from build123d import *

# Parameters (mm, degrees)
BOSS_EXTRUDE1_DEPTH = 100


with BuildPart() as part:
    # Sketch1 → Boss-Extrude1 (new body)
    with BuildSketch(Plane.XY):
        with BuildLine():
            Line((0, 0), (11, 0))
            Line((11, 0), (11, -0.9))
            Line((11, -0.9), (9.5, -0.9))
            ThreePointArc((9.5, -0.9), (9.128025612, -1.798025612), (8.23, -2.17))
            Line((8.23, -2.17), (8.23, -3.07))
            Line((8.23, -3.07), (12.415281374, -3.07))
            Line((12.415281374, -3.07), (13.949747468, -1.535533906))
            Line((13.949747468, -1.535533906), (10.414213562, 2))
            Line((10.414213562, 2), (0.585786438, 2))
            Line((0.585786438, 2), (-2.814747468, -1.400533906))
            Line((-2.814747468, -1.400533906), (-1.145281374, -3.07))
            Line((-1.145281374, -3.07), (2.77, -3.07))
            Line((2.77, -3.07), (2.77, -2.17))
            ThreePointArc((2.77, -2.17), (1.871974388, -1.798025612), (1.5, -0.9))
            Line((1.5, -0.9), (0, -0.9))
            Line((0, -0.9), (0, 0))
        make_face()
    extrude(amount=BOSS_EXTRUDE1_DEPTH)


solid = part.part
Geometry: final body of the model. Coordinates: model frame, mm. Round coordinates to 2 decimals unless told otherwise and drop trailing zeros. Loops run counter-clockwise (first coordinate to the right, second up) from the corner with the lowest first, then second, coordinate; pieces in that order, holes last.
Q1. Material intervals for L1, parallel to Y at x = 3.5, z = 46; L2, parallel to X at y = -0.75, z = 58; L3, parallel to X at y = -2.65, z = 77, sorted ascending.
Q2. Pin query (flat end, axial travel): P1, Ø1, axis at x = 7.5, z = 67.5, coming from the -Y side; P2, Ø0.7, axis at y = -2.5, z = 74.5, coming from the -X side; P3, Ø1.5, axis at y = -2.5, z = 83, coming from the +X side. Return the tip coordinate at first contact, or that it passes through.
Q3. Section A-A on z = 9. Return loops of the section in (x, y).
Q4. Section B-B on x = 5.25. Return loops of the section in (y, z), plus the area to 3 significant figures.
Q5. Section C-C on y = 0.8. Return loops of the section in (x, z), plus the area to 3 significant figures.
Q6. Pull-direction query (Y, two-part tool) for faces 1 (the flat face through (5, 1, 100)), 2 (the flat face through (13.172, -2.314, 49.3)), 3 (the flat face through (-1.091, 0.324, 49.3)), 4 (the flat face through (5, 0, 49)); classes: released by +Y, released by -Y, zero draft, split by the parting line, or undercut.
Evaluation:
1. L1: y = 0 to 2
1. L2: x = -2.16 to 0, 11 to 13.16
1. L3: x = -1.57 to 2.77, 8.23 to 12.84
2. P1: stops at y = 0
2. P2: stops at x = -2.07
2. P3: stops at x = 13.74
3. outline: (-2.81, -1.4) - (-1.15, -3.07) - (2.77, -3.07) - (2.77, -2.17) arc R1.27 cw to (1.5, -0.9) - (0, -0.9) - (0, 0) - (11, 0) - (11, -0.9) - (9.5, -0.9) arc R1.27 cw to (8.23, -2.17) - (8.23, -3.07) - (12.42, -3.07) - (13.95, -1.54) - (10.41, 2) - (0.59, 2) - close
4. outline: (0, 0) - (2, 0) - (2, 100) - (0, 100) - close
4. area: 200 mm2
5. outline: (-0.61, 0) - (11.61, 0) - (11.61, 100) - (-0.61, 100) - close
5. area: 1,220 mm2
6. face 1: zero draft
6. face 2: released by -Y
6. face 3: released by +Y
6. face 4: undercut
